Answer from the drawing. Dimensions are ordinates in mm from the lowest x, y and z of the part. A direction names the side the tool comes from. Coordinates: 2 decimals unless noted, no trailing zeros. Order: outer loops, then holes, each group sorted by start corner. A loop starts at its lowest first (then second) coordinate and runs counter-clockwise, first axis right, second up. Notation, with made-up numbers: (-37.5, -26.5) -> (-21.5, -26.5) arc R19 cw to (-21.5, -12.5) -> close; hole circle Ø4 at (62.25, -11). An arc over 180 degrees is marked (long way). Answer in a Markdown table with one row per item.
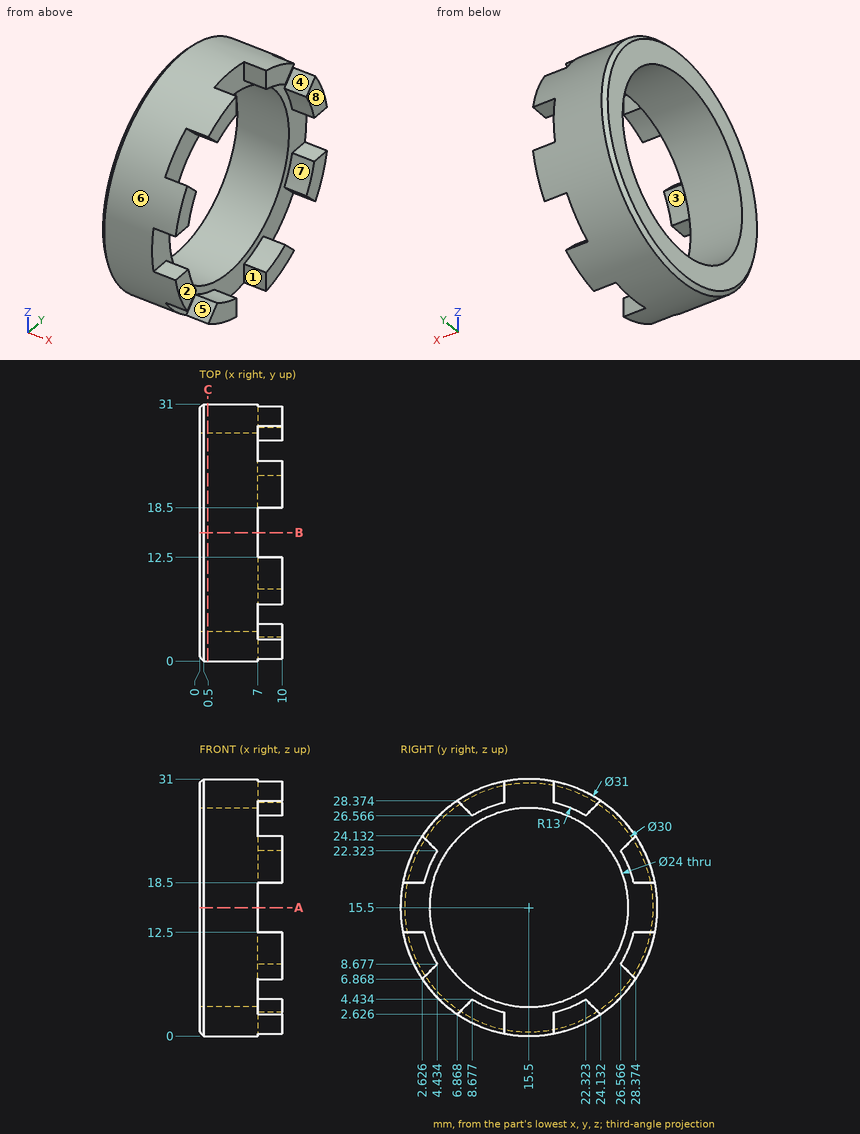
Q1. Given pin 1 (0.8 mm diameter, centred on x = 8.5, y = 29, fed in from +Z) (1 decimal); pin 2 (3 mm diameter, centred on x = 9, z = 29, fed in from -Y); pin 3 (3 mm diameter, centred on x = 8.5, y = 29, fed in from -Z); pin 4 (12 mm diameter, centred on y = 4, z = 26, fed in from -X), each flat-ended and moving along its own axis, determine where each tip first touches the part or whether it passes through.
Outcome:
| item | result |
|---|---|
| pin 1 | z = 23.8 |
| pin 2 | y = 6.87 |
| pin 3 | z = 6.87 |
| pin 4 | x = 0 |
Q2. For the marked faces 1, 2, 3, 4 and 5, determine the directions among +Z, -Z, +X, -X, +Y, -Y from which every point of the face is accessible in a straight line to the end or side of a thin tool.
Outcome:
| item | result |
|---|---|
| face 1 | +Z, -Z, +X |
| face 2 | +Z, -Z, +X, +Y, -Y |
| face 3 | +X |
| face 4 | +Z, +X |
| face 5 | +X, -Y |
Q3. The part is cut by section C-C (x = 1). Write down the section's boundary in (y, z).
Outcome:
| item | result |
|---|---|
| outline | circle Ø31 at (15.5, 15.5); hole circle Ø24 at (15.5, 15.5) |
Q4. Consider line 1 (Y direction, x = 5, z = 15.5); line 2 (Y direction, x = 1.5, z = 21) (1 decimal); line 3 (Z direction, x = 3, y = 19). Determine where each line is inside the solid, lowest interval first.
Outcome:
| item | result |
|---|---|
| line 1 | 0 to 3.5, 27.5 to 31 |
| line 2 | 1 to 4.8, 26.2 to 30 |
| line 3 | 0.4 to 4.02, 26.98 to 30.6 |
Q5. The part is cut by section A-A (z = 15.5). Write down the section's boundary in (x, y).
Outcome:
| item | result |
|---|---|
| outline | (0, 0.5) -> (0.5, 0) -> (7, 0) -> (7, 3.5) -> (0, 3.5) -> close; (0, 27.5) -> (7, 27.5) -> (7, 31) -> (0.5, 31) -> (0, 30.5) -> close |
Q6. For a pull along Z with two mould halves and no side action, classify the marked faces 6, 7 and 8 as pulls with the +Z half, pulls with the -Z half, needs draft (parallel to the pull), parting line crosses it, or undercut.
Outcome:
| item | result |
|---|---|
| face 6 | parting line crosses it |
| face 7 | undercut |
| face 8 | needs draft |
